Design review of the part built by this model. Coordinates are the model's own, in mm. Face numbers are marked on the shaded views. Coordinates: 2 decimals unless noted, no trailing zeros. Loops run counter-clockwise (first coordinate to the right, second up) from the corner with the lowest first, then second, coordinate; pieces in that order, holes last.
from build123d import *

# Parameters (mm, degrees)
SKIZZE1_W                       = 45
SKIZZE1_H                       = 30
SKIZZE1_R                       = 11.85
SKIZZE1_R_2                     = 1.75
AUFSATZ_LINEAR_AUSTRAGEN1_DEPTH = 9
SKIZZE3_R                       = 12.85
SCHNITT_LINEAR_AUSTRAGEN1_DEPTH = 7


with BuildPart() as part:
    # Skizze1 → Aufsatz-Linear austragen1 (new body)
    with BuildSketch(Plane.XY):
        Rectangle(SKIZZE1_W, SKIZZE1_H)
        Circle(SKIZZE1_R, mode=Mode.SUBTRACT)
        with Locations((-17.5, 0)):
            Circle(SKIZZE1_R_2, mode=Mode.SUBTRACT)
        with Locations((17.5, 0)):
            Circle(SKIZZE1_R_2, mode=Mode.SUBTRACT)
    extrude(amount=AUFSATZ_LINEAR_AUSTRAGEN1_DEPTH)

    # Skizze3 → Schnitt-Linear austragen1 (cut)
    with BuildSketch(Plane.XY.offset(9)):
        Circle(SKIZZE3_R)
    extrude(amount=-SCHNITT_LINEAR_AUSTRAGEN1_DEPTH, mode=Mode.SUBTRACT)


solid = part.part
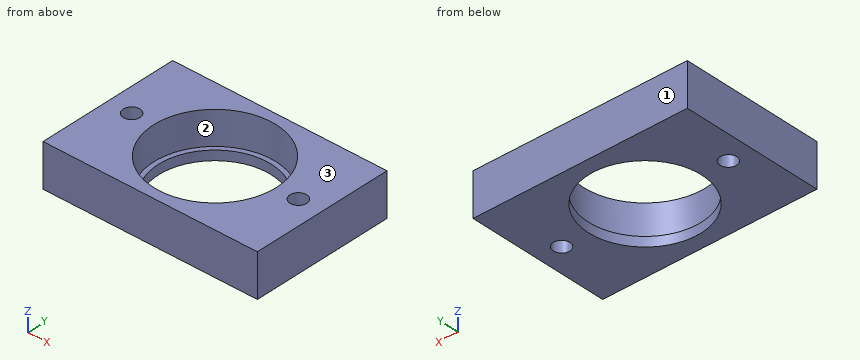
Q1. Take a section at B-B, the plane z = 3. Write out the cut boundary in (x, y).
Q2. Take a section at A-A, the plane x = -17.5. Write out the cut boundary in (y, z), then the cut area to 4 significant figures.
Q3. Take a section at C-C, the plane y = 4.5. Write out the cut boundary in (x, z), then the cut area to 3 significant figures.
Q4. Take a section at D-D, the plane y = 0. Write out the cut boundary in (x, z).
Q5. For line 1 (Y direction, x = 0, z = 4.25); line 2 (Y direction, x = -17.5, z = 6); line 3 (X direction, y = 7, z = 2.25), list the stretches that pass through material, from the lowest coordinate up.
Q6. The part is to be moulded in two halves that separate along Y. For the marked faces 1, 2 and 3, say which applies: pulls with the +Y half, pulls with the -Y half, needs draft (parallel to the pull), parting line crosses it, or undercut.
Q7. Clearance check with a flat-ended pin moving along its axis: pin 1 Ø6 at (x, y) = (-15.5, -11.5) entering from -Z. State where the tip first meets the part, or that it passes through.
Entries:
1. outline: (-22.5, -15) - (22.5, -15) - (22.5, 15) - (-22.5, 15) - close; hole circle Ø3.5 at (-17.5, 0); hole circle Ø25.7 at (0, 0); hole circle Ø3.5 at (17.5, 0)
2. outline: (-15, 0) - (-1.75, 0) - (-1.75, 9) - (-15, 9) - close; (1.75, 0) - (15, 0) - (15, 9) - (1.75, 9) - close
2. area: 238.5 mm2
3. outline: (-22.5, 0) - (-10.96, 0) - (-10.96, 2) - (-12.04, 2) - (-12.04, 9) - (-22.5, 9) - close; (10.96, 0) - (22.5, 0) - (22.5, 9) - (12.04, 9) - (12.04, 2) - (10.96, 2) - close
3. area: 193 mm2
4. outline: (-22.5, 0) - (-19.25, 0) - (-19.25, 9) - (-22.5, 9) - close; (-15.75, 0) - (-11.85, 0) - (-11.85, 2) - (-12.85, 2) - (-12.85, 9) - (-15.75, 9) - close; (11.85, 0) - (15.75, 0) - (15.75, 9) - (12.85, 9) - (12.85, 2) - (11.85, 2) - close; (19.25, 0) - (22.5, 0) - (22.5, 9) - (19.25, 9) - close
5. line 1: y = -15 to -12.85, 12.85 to 15
5. line 2: y = -15 to -1.75, 1.75 to 15
5. line 3: x = -22.5 to -10.78, 10.78 to 22.5
6. face 1: pulls with the +Y half
6. face 2: undercut
6. face 3: needs draft
7. pin 1: stops at z = 0
